from build123d import *

# Parameters (mm, degrees)
BOSS_EXTRUDE1_DEPTH = 1
BOSS_EXTRUDE2_DEPTH = 1.5


with BuildPart() as part:
    # Sketch1 → Boss-Extrude1 (new body)
    with BuildSketch(Plane.XY):
        Polygon((-85, 42), (85, 42), (86.5, 0), (85, -42), (-85, -42), (-86.5, 0), align=None)
    extrude(amount=BOSS_EXTRUDE1_DEPTH)

    # Sketch2 → Boss-Extrude2 (add)
    with BuildSketch(Plane.XY.offset(1)):
        Polygon((-83, 40.25), (83, 40.25), (84.5, 0), (83, -40.25), (-83, -40.25), (-84.5, 0), align=None)
    extrude(amount=BOSS_EXTRUDE2_DEPTH)


solid = part.part
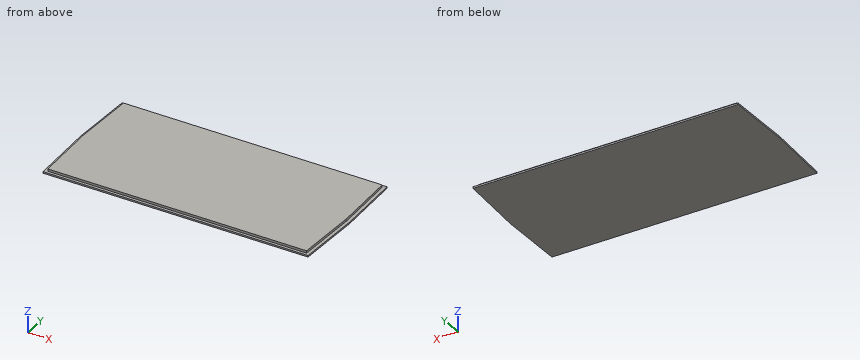
The listing builds one solid part. Answer for the finished solid, in the listing's coordinates (mm). Round coordinates to 2 decimals unless told otherwise and drop trailing zeros. Write each loop counter-clockwise with the first axis right and the second up, starting at its lowest first coordinate (ties: lowest second). Pieces come first, ordered by that corner, then holes. Notation, with made-up numbers: M 70.5,-18.5 L 110.5,-18.5 A35 cw 110.5,15.5 Z; hole C 56.25,79 d6. An arc over 180 degrees is marked long. Write each question's results on one line, items separated by ' | '. Start each with the question number.
(1) The part is cut by section C-C, the plane z = 2. Write down the section's boundary in (x, y).
(2) The part is cut by section A-A, the plane x = -55.5. Write down the section's boundary in (y, z).
(3) The part is cut by section B-B, the plane y = -32.5. Write down the section's boundary in (x, z).
(4) Find the intervals of material crossed by line 1 (Y direction, x = 58, z = 1.3); line 2 (X direction, y = 16, z = 0.85); line 3 (X direction, y = 11.5, z = 1.5), in increasing order.
(5) Each of these flat-tipped pins is pushed along its axis until it touches: P1, Ø1.2, axis at x = 30, z = 2, coming from the -Y side; P2, Ø1, axis at y = 22.5, z = 1, coming from the +X side; P3, Ø1, axis at y = 5.5, z = 1, coming from the +X side. Where does it stop, or does it pass through?
Worked answers:
1) outline: M -84.5,0 L -83,-40.25 L 83,-40.25 L 84.5,0 L 83,40.25 L -83,40.25 Z
2) outline: M -42,0 L 42,0 L 42,1 L 40.25,1 L 40.25,2.5 L -40.25,2.5 L -40.25,1 L -42,1 Z
3) outline: M -85.34,0 L 85.34,0 L 85.34,1 L 83.29,1 L 83.29,2.5 L -83.29,2.5 L -83.29,1 L -85.34,1 Z
4) line 1: y = -40.25 to 40.25 | line 2: x = -85.93 to 85.93 | line 3: x = -84.07 to 84.07
5) P1: stops at y = -40.25 | P2: stops at x = 85.71 | P3: stops at x = 86.32
